Source: CAD feature listing. Evaluate the final solid. Frame: model axes, mm. Face numbers are marked on the shaded views. A direction names the side the tool comes from. Give positions to 0.01 mm unless a question says otherwise; leave off trailing zeros. Order: outer loops, then holes, each group sorted by start corner. A loop starts at its lowest first (then second) coordinate and runs counter-clockwise, first axis right, second up. Notation, with made-up numbers: M 43,3 L 62,3 A29 ccw 62,25 Z; hole C 87.5,-35 d7. An arc over 180 degrees is marked long. Return JSON: item names as keys, results as strings.
from build123d import *

# Parameters (mm, degrees)
SKETCH3_R          = 25
CUT_EXTRUDE1_DEPTH = 10
SKETCH5_R          = 25
CUT_EXTRUDE2_DEPTH = 36


with BuildPart() as part:
    # Sketch2 → Revolve1 (revolve)
    with BuildSketch(Plane.XY, mode=Mode.PRIVATE) as revolve1_sk:
        Polygon((0, 0), (52, 0), (52, 8), (40.216748768, 8), (40.216748768, 28), (52, 28), (52, 36), (0, 36), align=None)
    revolve(revolve1_sk.sketch.rotate(Axis((0, 36, 0), (0, -1, 0)), 180), axis=Axis((0, 36, 0), (0, -1, 0)))

    # Sketch3 → Cut-Extrude1 (cut)
    with BuildSketch(Plane(origin=(0, 36, 0), x_dir=(1, 0, 0), z_dir=(0, 1, 0))):
        with Locations(Location((0, 0, 0), (0, 0, 180))):
            Circle(SKETCH3_R)
    extrude(amount=-CUT_EXTRUDE1_DEPTH, mode=Mode.SUBTRACT)

    # Sketch5 → Cut-Extrude2 (cut)
    with BuildSketch(Plane(origin=(0, 26, 0), x_dir=(1, 0, 0), z_dir=(0, 1, 0))):
        with Locations(Location((0, 0, 0), (0, 0, 180))):
            Circle(SKETCH5_R)
    extrude(amount=-CUT_EXTRUDE2_DEPTH, mode=Mode.SUBTRACT)


solid = part.part
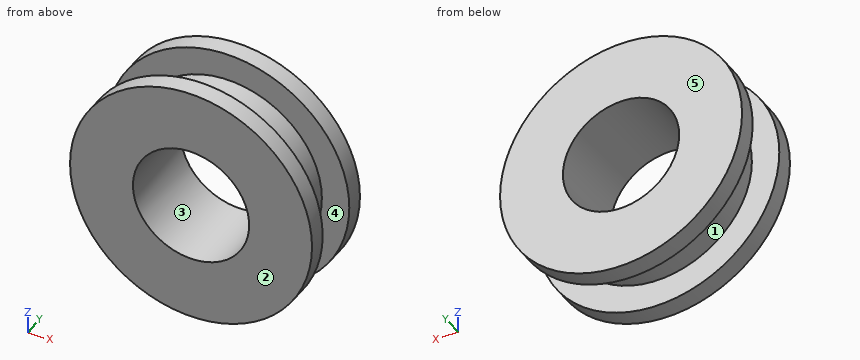
1. Section query B-B (x = 0). Return loops of the section in (y, z), then the cut area to 3 significant figures.
Evaluation:
{"outline": "M 0,-52 L 8,-52 L 8,-40.22 L 28,-40.22 L 28,-52 L 36,-52 L 36,-25 L 0,-25 Z; M 0,25 L 36,25 L 36,52 L 28,52 L 28,40.22 L 8,40.22 L 8,52 L 0,52 Z", "area": "1,470 mm^2"}
2. First-contact query: pin 1 (12 mm diameter, centred on x = 19.5, y = 20.5, fed in from -Z); pin 2 (3 mm diameter, centred on x = -8, y = 4, fed in from -Z); pin 3 (1.5 mm diameter, centred on x = -20.5, y = 9.5, fed in from +Z); pin 4 (8 mm diameter, centred on x = 10, z = 17.5, fed in from +Y). Flat tips, straight axial feed; report the tip coordinate or a pass-through.
Evaluation:
{"pin 1": "stops at z = -37.88", "pin 2": "stops at z = -51.59", "pin 3": "stops at z = 35.03", "pin 4": "passes through"}
3. Section query C-C (y = 30). Return loops of the section in (x, z).
Evaluation:
{"outline": "C 0,0 d104; hole C 0,0 d50"}
4. Draft query along Y for the marked faces 1, 2 and 3. Return one class per face: pulls with the +Y half, pulls with the -Y half, needs draft (parallel to the pull), parting line crosses it, or undercut.
Evaluation:
{"face 1": "undercut", "face 2": "pulls with the -Y half", "face 3": "needs draft"}
5. Ray query, probe 1 along Y at (x, z) = (46, 15); probe 2 along Z at (x, y) = (0, 13); probe 3 along Z at (x, y) = (-14, 10.5). Return the intervals inside material, ascending.
Evaluation:
{"probe 1": "y = 0 to 8, 28 to 36", "probe 2": "z = -40.22 to -25, 25 to 40.22", "probe 3": "z = -37.7 to -20.71, 20.71 to 37.7"}
6. Section query D-D (x = -30). Return loops of the section in (y, z).
Evaluation:
{"outline": "M 0,-42.47 L 8,-42.47 L 8,-26.78 L 28,-26.78 L 28,-42.47 L 36,-42.47 L 36,42.47 L 28,42.47 L 28,26.78 L 8,26.78 L 8,42.47 L 0,42.47 Z"}
7. Section query A-A (z = 0). Return loops of the section in (x, y), then the cut area to 3 significant figures.
Evaluation:
{"outline": "M -52,0 L -25,0 L -25,36 L -52,36 L -52,28 L -40.22,28 L -40.22,8 L -52,8 Z; M 25,0 L 52,0 L 52,8 L 40.22,8 L 40.22,28 L 52,28 L 52,36 L 25,36 Z", "area": "1,470 mm^2"}
8. Set-up query: the marked faces 4 and 5. Return all of +Z, -Z, +X, -X, +Y, -Y with unobstructed straight access to the full face (end or side cutting, diameter ignored); none if empty.
Evaluation:
{"face 4": "none", "face 5": "+Z, -Z, +X, -X, +Y"}
